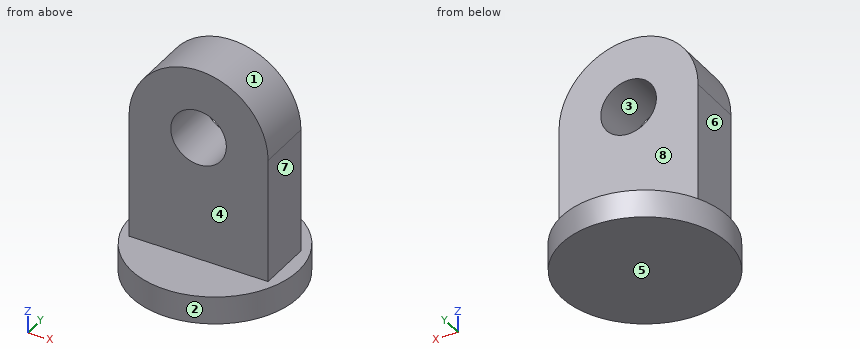
from build123d import *

# Parameters (mm, degrees)
F0_R     = 3
F1_DEPTH = 1
F2_W     = 5
F2_H     = 2
F3_DEPTH = 4.5
F5_DEPTH = 1
F6_R     = 1
F7_DEPTH = 25


with BuildPart() as f1:
    # F0 (on Top) → F1 (new body)
    with BuildSketch(Plane.XY):
        Circle(F0_R)
    extrude(amount=F1_DEPTH)

    # F2 (on face) → F3 (join)
    with BuildSketch(Plane.XY.offset(1)):
        Rectangle(F2_W, F2_H)
    extrude(amount=F3_DEPTH)

    # F4 (on Front) → F5 (join, symmetric)
    with BuildSketch(Plane.XZ):
        with BuildLine():
            Line((0, 5.5), (2.5, 5.5))
            ThreePointArc((2.5, 5.5), (0, 8), (-2.5, 5.5))
            Line((-2.5, 5.5), (0, 5.5))
        make_face()
    extrude(amount=F5_DEPTH, both=True)

    # F6 (on face) → F7 (cut)
    with BuildSketch(Plane.XZ.offset(1)):
        with Locations((0, 5.5)):
            Circle(F6_R)
    extrude(amount=-F7_DEPTH, mode=Mode.SUBTRACT)


solid = f1.part
Check sheet for the modelled part. Datum: model origin and axes. Units: mm. Face numbers are marked on the shaded views. A direction names the side the tool comes from. Round coordinates to 2 decimals unless told otherwise and drop trailing zeros. Write each loop counter-clockwise with the first axis right and the second up, starting at its lowest first coordinate (ties: lowest second). Pieces come first, ordered by that corner, then holes. Notation, with made-up numbers: (28.25, 44) -> (58.25, 44) arc R12 ccw to (58.25, 57) -> close; hole circle Ø1 at (67.25, 1.5). An arc over 180 degrees is marked (long way). Answer as CSV lines item,"result". Start each with the question number.
1) Go/stop test with flat-tipped pins: P1, Ø1.5, axis at x = 2, z = 2, coming from the +Y side; P2, Ø1, axis at y = 0.5, z = 2, coming from the +X side; P3, Ø2, axis at y = -0.5, z = 6.5, coming from the -X side. Record where each tip stops, or that it passes through.
2) Release check for a two-part mould opening along Z. For the marked faces 1, 2 and 3 record: pulls with the +Z half, pulls with the -Z half, needs draft (parallel to the pull), parting line crosses it, or undercut.
3) Section check A-A on x = 0. Enter the section's corners in (y, z), and give its area (3 significant figures).
4) Section check D-D on z = 1.75. Enter the section's corners in (x, y).
5) Tool access check on the marked faces 4, 5, 6, 7 and 8. Record the directions out of +Z, -Z, +X, -X, +Y, -Y that give a thin tool (end or side, any length) a straight path to the whole face; none if there is none.
6) Material ranges on line 1 (Z direction, x = 0, y = -0.25); line 2 (X direction, y = 0, z = 4); line 3 (Z direction, x = -0.9, y = -1.3), recorded low to high. Write a range as from..to.
7) Section check B-B on z = 5.25. Enter the section's corners in (x, y).
8) Section check C-C on y = 0.2. Enter the section's corners in (x, z).
Found:
1,P1,"stops at y = 1"
1,P2,"stops at x = 2.5"
1,P3,"stops at x = -2.5"
2,face 1,"pulls with the +Z half"
2,face 2,"needs draft"
2,face 3,"undercut"
3,outline,"(-3, 0) -> (3, 0) -> (3, 1) -> (1, 1) -> (1, 4.5) -> (-1, 4.5) -> (-1, 1) -> (-3, 1) -> close; (-1, 6.5) -> (1, 6.5) -> (1, 8) -> (-1, 8) -> close"
3,area,"16.0 mm^2"
4,outline,"(-2.5, -1) -> (2.5, -1) -> (2.5, 1) -> (-2.5, 1) -> close"
5,face 4,"+Z, +X, -X, -Y"
5,face 5,"-Z, +X, -X, +Y, -Y"
5,face 6,"+Z, -X, +Y, -Y"
5,face 7,"+Z, +X, +Y, -Y"
5,face 8,"+Z, +X, -X, +Y"
6,line 1,"z = 0..4.5, 6.5..8"
6,line 2,"x = -2.5..2.5"
6,line 3,"z = 0..1"
7,outline,"(-2.5, -1) -> (-0.97, -1) -> (-0.97, 1) -> (-2.5, 1) -> close; (0.97, -1) -> (2.5, -1) -> (2.5, 1) -> (0.97, 1) -> close"
8,outline,"(-2.99, 0) -> (2.99, 0) -> (2.99, 1) -> (2.5, 1) -> (2.5, 5.5) arc R2.5 ccw to (-2.5, 5.5) -> (-2.5, 1) -> (-2.99, 1) -> close; hole circle Ø2 at (0, 5.5)"
